```python
from build123d import *

# Parameters (mm, degrees)
F0_W        = 101.6
F0_H        = 152.4
F1_DEPTH    = 95.25
F2_T1_DEPTH = 443.6748663003
F4_DEPTH    = 59.944


# Not quite as in the source:
# - a fillet or chamfer that OpenCascade refuses, or shapes differently, is made with other operations: its cross-section is extruded or revolved along the edge and cut away or added


with BuildPart() as f1:
    # F0 (on Top) → F1 (new body)
    with BuildSketch(Plane.XY):
        with Locations((2.2735033583, 3.7213955075)):
            Rectangle(F0_W, F0_H)
    extrude(amount=F1_DEPTH)

    # F2: fillet of radius 58.2549732601 on 2 edges, made by hand

    # F2_s2 → F2_t1 (cut)
    with BuildSketch(Plane.XZ.offset(-225.5588286576)):
        with BuildLine():
            ThreePointArc((-48.5264966417, 58.2549732601), (-31.4640100116, 17.06248663), (9.7284766184, 0))
            Line((9.7284766184, 0), (-48.5264966417, 0))
            Line((-48.5264966417, 0), (-48.5264966417, 58.2549732601))
        make_face()
        with BuildLine():
            ThreePointArc((53.0735033583, 58.2549732601), (36.0110167283, 17.06248663), (-5.1814699017, 0))
            Line((-5.1814699017, 0), (53.0735033583, 0))
            Line((53.0735033583, 0), (53.0735033583, 58.2549732601))
        make_face()
    extrude(amount=F2_T1_DEPTH, mode=Mode.SUBTRACT)

    # F3 (on face) → F4 (cut)
    with BuildSketch(Plane.XY.offset(95.25)):
        Polygon((-40.9064966417, 17.4030140042), (-40.9064966417, -64.8586044925), (45.4535033583, -64.8586044925), (45.4535033583, 17.9895181209), (45.4535033583, 72.3013955075), (-40.9064966417, 72.3013955075), align=None)
    extrude(amount=-F4_DEPTH, mode=Mode.SUBTRACT)


solid = f1.part
```
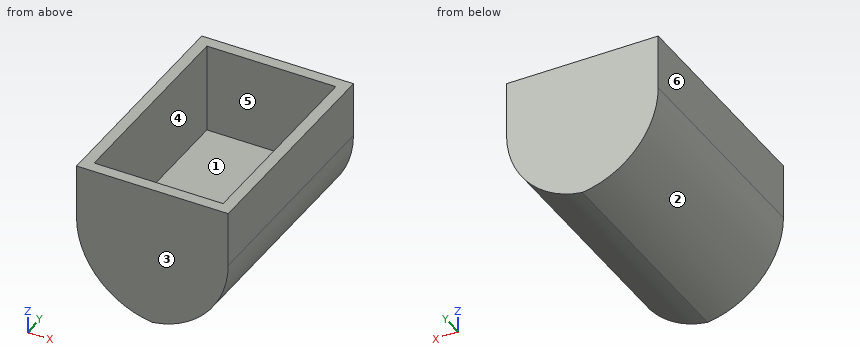
Input: part model. Units: mm. Frame: model coordinates. Face numbers are marked on the shaded views. A direction names the side the tool comes from. Give positions to 0.01 mm unless a question says otherwise; leave off trailing zeros. Loops run counter-clockwise (first coordinate to the right, second up) from the corner with the lowest first, then second, coordinate; pieces in that order, holes last.
1) Section query A-A on z = 71. Return the cut outline in (x, y).
A:
outline: (-48.53, -72.48) - (53.07, -72.48) - (53.07, 79.92) - (-48.53, 79.92) - close; hole (-40.91, -64.86) - (45.45, -64.86) - (45.45, 72.3) - (-40.91, 72.3) - close
2) Contact query for flat-ended pins moving along their axis: pin 1 (2 mm diameter, centred on x = -14.5, y = -45.5, fed in from -Z); pin 2 (1 mm diameter, centred on y = 39, z = 36, fed in from -X); pin 3 (3 mm diameter, centred on x = -33, y = -17, fed in from -Z). Output: stop coordinate, or through.
A:
pin 1: stops at z = 4.83
pin 2: stops at x = -44.31
pin 3: stops at z = 17.1
3) Section query C-C on x = 10.5. Return the cut outline in (y, z).
A:
outline: (-72.48, 2.15) - (79.92, 2.15) - (79.92, 95.25) - (72.3, 95.25) - (72.3, 35.31) - (-64.86, 35.31) - (-64.86, 95.25) - (-72.48, 95.25) - close
4) Reachability of the marked faces 5 and 6 from +Z, -Z, +X, -X, +Y, -Y: full face, straight path, thin tool, end or side. Return the list, or none.
A:
face 5: +Z
face 6: +Z, -Z, -X, +Y, -Y
5) Section query B-B on y = 53. Return the cut outline in (x, z).
A:
outline: (-48.53, 58.25) arc R58.25 ccw to (2.27, 0.48) arc R58.25 ccw to (53.07, 58.25) - (53.07, 95.25) - (45.45, 95.25) - (45.45, 35.31) - (-40.91, 35.31) - (-40.91, 95.25) - (-48.53, 95.25) - close
6) Line query: L1, parallel to Y at x = -38.5, z = 56; L2, parallel to X at y = 59, z = 86.5; L3, parallel to X at y = 13, z = 51.5. Output: solid intervals per line, ascending.
A:
L1: y = -72.48 to -64.86, 72.3 to 79.92
L2: x = -48.53 to -40.91, 45.45 to 53.07
L3: x = -48.13 to -40.91, 45.45 to 52.68
7) Section query D-D on z = 52.5. Return the cut outline in (x, y).
A:
outline: (-48.24, -72.48) - (52.79, -72.48) - (52.79, 79.92) - (-48.24, 79.92) - close; hole (-40.91, -64.86) - (45.45, -64.86) - (45.45, 72.3) - (-40.91, 72.3) - close
8) Mould query, pull axis Y, two halves, no side actions, for the marked faces 1, 2, 3 and 4. Classes: released by +Y, released by -Y, zero draft, split by the parting line, or undercut.
A:
face 1: undercut
face 2: zero draft
face 3: released by -Y
face 4: undercut
